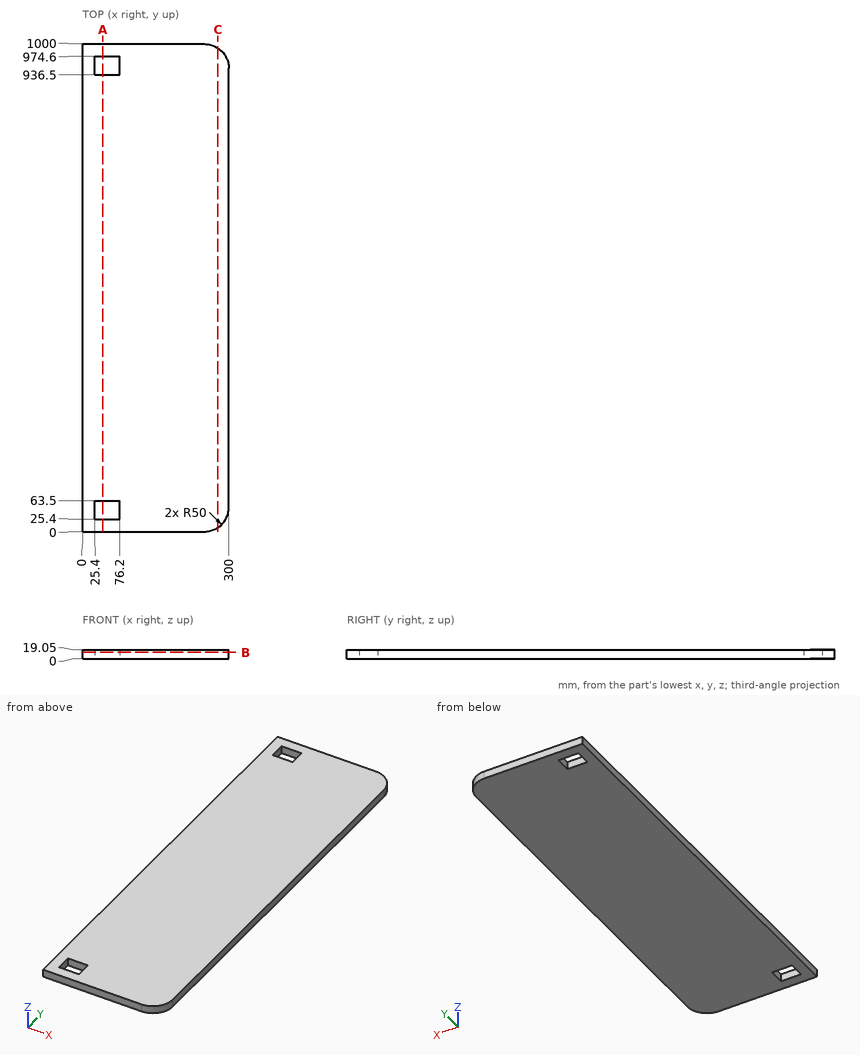
For this review, use the dimensioned drawing (mm, ordinates from the lowest corner) and the shaded views. Round coordinates to 2 decimals unless told otherwise and drop trailing zeros. Write each loop counter-clockwise with the first axis right and the second up, starting at its lowest first coordinate (ties: lowest second). Pieces come first, ordered by that corner, then holes. Notation, with made-up numbers: M -7,9.5 L 2,9.5 A30 cw 2,36.5 Z; hole C 84.25,28 d8. An arc over 180 degrees is marked long. Answer as CSV lines item,"result". Start each with the question number.
Q1. Consider section B-B, the plane z = 13.5. Give the boundary of the cut face in (x, y), then the cut area to 3 significant figures.
Q2. Consider section C-C, the plane x = 277.5. Give the boundary of the cut face in (y, z), then the cut area to 3 significant figures.
Q3. Wall thickness on line 1 along Y through (x, z) = (29.5, 6.5); line 2 along Y through (x, z) = (277, 7); line 3 along Y through (x, z) = (284.5, 7.75): over which ranges is each line inside the solid? List them lowest first.
Q4. Consider section A-A, the plane x = 42. Give the boundary of the cut face in (y, z), then the cut area to 3 significant figures.
Result set:
1,outline,"M 0,0 L 250,0 A50 ccw 300,50 L 300,950 A50 ccw 250,1000 L 0,1000 Z; hole M 25.4,25.4 L 76.2,25.4 L 76.2,63.5 L 25.4,63.5 Z; hole M 25.4,936.5 L 76.2,936.5 L 76.2,974.6 L 25.4,974.6 Z"
1,area,"295,000 mm²"
2,outline,"M 8.24,0 L 991.76,0 L 991.76,19.05 L 8.24,19.05 Z"
2,area,"18,700 mm²"
3,line 1,"y = 0 to 25.4, 63.5 to 936.5, 974.6 to 1000"
3,line 2,"y = 7.92 to 992.08"
3,line 3,"y = 13.81 to 986.19"
4,outline,"M 0,0 L 25.4,0 L 25.4,19.05 L 0,19.05 Z; M 63.5,0 L 936.5,0 L 936.5,19.05 L 63.5,19.05 Z; M 974.6,0 L 1000,0 L 1000,19.05 L 974.6,19.05 Z"
4,area,"17,600 mm²"
